from build123d import *

# Parameters (mm, degrees)
F0_R     = 10
F1_DEPTH = 10
F2_DEPTH = 47.5
F3_R     = 7.5
F4_DEPTH = 60.001
F5_R     = 17
F5_R_2   = 10
F6_DEPTH = 3


with BuildPart() as f1:
    # F0 (on Top) → F1 (new body)
    with BuildSketch(Plane.XY):
        with BuildLine():
            ThreePointArc((13.2287565553, -15), (18.2287565553, -8.2287565553), (20, 0))
            ThreePointArc((20, 0), (18.2287565553, 8.2287565553), (13.2287565553, 15))
            ThreePointArc((13.2287565553, 15), (0, 20), (-13.2287565553, 15))
            ThreePointArc((-13.2287565553, 15), (-18.2287565565, 8.2287565528), (-20, -5.5e-09))
            ThreePointArc((-20, -5.5e-09), (-18.2287565542, -8.2287565578), (-13.2287565553, -15))
            ThreePointArc((-13.2287565553, -15), (0, -20), (13.2287565553, -15))
        make_face()
        Circle(F0_R, mode=Mode.SUBTRACT)
        with BuildLine():
            ThreePointArc((13.2287565553, 15), (18.2287565553, 8.2287565553), (20, 0))
            Line((20, 0), (20, 15))
            Line((20, 15), (13.2287565553, 15))
        make_face()
        with BuildLine():
            Line((20, -15), (20, 0))
            ThreePointArc((20, 0), (18.2287565553, -8.2287565553), (13.2287565553, -15))
            Line((13.2287565553, -15), (20, -15))
        make_face()
        with BuildLine():
            Line((-20, -15), (-13.2287565553, -15))
            ThreePointArc((-13.2287565553, -15), (-18.2287565542, -8.2287565578), (-20, -5.5e-09))
            Line((-20, -5.5e-09), (-20, -15))
        make_face()
        with BuildLine():
            ThreePointArc((-20, -5.5e-09), (-18.2287565565, 8.2287565528), (-13.2287565553, 15))
            Line((-13.2287565553, 15), (-20, 15))
            Line((-20, 15), (-20, -5.5e-09))
        make_face()
    extrude(amount=F1_DEPTH)

    # F0 (on Top) → F2 (join)
    with BuildSketch(Plane.XY):
        Polygon((20, 15), (20, 0), (20, -15), (30, -15), (30, 15), align=None)
        Polygon((-20, -15), (-20, -5.5e-09), (-20, 15), (-30, 15), (-30, -15), align=None)
    extrude(amount=F2_DEPTH)

    # F3 (on face) → F4 (cut, through all)
    with BuildSketch(Plane.YZ.offset(30)):
        with BuildLine():
            Line((15, 47.5), (-15, 47.5))
            Line((-15, 47.5), (-15, 32))
            ThreePointArc((-15, 32), (0, 47), (15, 32))
            Line((15, 32), (15, 47.5))
        make_face()
        with Locations((0, 32)):
            Circle(F3_R)
    extrude(amount=-F4_DEPTH, mode=Mode.SUBTRACT)

    # F5 (on face) → F6 (join)
    with BuildSketch(Plane.XY):
        Circle(F5_R)
        Circle(F5_R_2, mode=Mode.SUBTRACT)
    extrude(amount=-F6_DEPTH)


solid = f1.part
Could you check a few things on this model? Use its own coordinates, in mm. A direction names the side the tool comes from. Coordinates: 2 decimals unless noted, no trailing zeros. Loops run counter-clockwise (first coordinate to the right, second up) from the corner with the lowest first, then second, coordinate; pieces in that order, holes last. Notation, with made-up numbers: (-7.75, 8) -> (40.25, 8) arc R37 ccw to (40.25, 45) -> close; hole circle Ø2 at (-16, 89). An arc over 180 degrees is marked (long way). Answer in a Markdown table with one row per item.
(1) Will these pins go through, and if not, where does the flat tip stop? pin 1 Ø12 at (x, y) = (0, 0) entering from +Z; pin 2 Ø24 at (y, z) = (0, 32) entering from -X; pin 3 Ø13.5 at (x, z) = (23, 18.5) entering from -Y; pin 4 Ø10 at (x, y) = (5, -5.5) entering from +Z.
Results found:
| item | result |
|---|---|
| pin 1 | passes through |
| pin 2 | stops at x = -30 |
| pin 3 | stops at y = -15 |
| pin 4 | stops at z = 10 |
(2) Imagine slicing it at C-C (z = 20). List the corners of the cut face in (x, y) for me.
Results found:
| item | result |
|---|---|
| outline | (-30, -15) -> (-20, -15) -> (-20, 15) -> (-30, 15) -> close; (20, -15) -> (30, -15) -> (30, 15) -> (20, 15) -> close |
(3) Imagine slicing it at D-D (x = 0). List the corners of the cut face in (y, z) for me, plus the area to 3 significant figures.
Results found:
| item | result |
|---|---|
| outline | (-20, 0) -> (-17, 0) -> (-17, -3) -> (-10, -3) -> (-10, 10) -> (-20, 10) -> close; (10, -3) -> (17, -3) -> (17, 0) -> (20, 0) -> (20, 10) -> (10, 10) -> close |
| area | 242 mm^2 |
(4) If I drill on probe 1 along Z at (x, y) = (-21.75, 0); probe 2 along X at (y, z) = (-7, 21); probe 3 along Y at (x, z) = (0, 6), over which ranges is the centre line in solid material (lowest first)?
Results found:
| item | result |
|---|---|
| probe 1 | z = 0 to 24.5, 39.5 to 47 |
| probe 2 | x = -30 to -20, 20 to 30 |
| probe 3 | y = -20 to -10, 10 to 20 |
(5) For faces 4 (the face through (23, -15, 12)), 5 (the face through (-9, 5, 10)), 6 (the face through (-23, 15, 12)), 7 (the face through (-24, -15, 12)), 8 (the face through (-0.4, -17.5, 0)), which set-ups out of +Z, -Z, +X, -X, +Y, -Y let a thin tool reach every point of the face, with its end or its side?
Results found:
| item | result |
|---|---|
| face 4 | +Z, -Z, +X, -Y |
| face 5 | +Z, +Y, -Y |
| face 6 | +Z, -Z, -X, +Y |
| face 7 | +Z, -Z, -X, -Y |
| face 8 | -Z |
(6) Thinking about a two-plate mould opening in X: for faces 1 (the face through (9.139, 14.334, -1.479)), 2 (the face through (20, 0, 24)), 3 (the face through (7.3, -7.3, -3)), which applies, released by +X, released by -X, zero draft, split by the parting line, or undercut?
Results found:
| item | result |
|---|---|
| face 1 | split by the parting line |
| face 2 | undercut |
| face 3 | zero draft |
(7) Imagine slicing it at A-A (z = 26). List the corners of the cut face in (x, y) for me.
Results found:
| item | result |
|---|---|
| outline | (-30, -15) -> (-20, -15) -> (-20, -4.5) -> (-30, -4.5) -> close; (-30, 4.5) -> (-20, 4.5) -> (-20, 15) -> (-30, 15) -> close; (20, -15) -> (30, -15) -> (30, -4.5) -> (20, -4.5) -> close; (20, 4.5) -> (30, 4.5) -> (30, 15) -> (20, 15) -> close |
(8) Imagine slicing it at B-B (y = 0). List the corners of the cut face in (x, z) for me, plus the area to 3 significant figures.
Results found:
| item | result |
|---|---|
| outline | (-30, 0) -> (-17, 0) -> (-17, -3) -> (-10, -3) -> (-10, 10) -> (-20, 10) -> (-20, 24.5) -> (-30, 24.5) -> close; (-30, 39.5) -> (-20, 39.5) -> (-20, 47) -> (-30, 47) -> close; (10, -3) -> (17, -3) -> (17, 0) -> (30, 0) -> (30, 24.5) -> (20, 24.5) -> (20, 10) -> (10, 10) -> close; (20, 39.5) -> (30, 39.5) -> (30, 47) -> (20, 47) -> close |
| area | 882 mm^2 |
